The listing builds one solid part. Answer for the finished solid, in the listing's coordinates (mm). Give positions to 0.01 mm unless a question says otherwise; leave off trailing zeros. Loops run counter-clockwise (first coordinate to the right, second up) from the corner with the lowest first, then second, coordinate; pieces in that order, holes last. Notation, with made-up numbers: M -29,14 L -4,14 A10 cw -4,33 Z; hole C 67.5,43.5 d5. An arc over 180 degrees is marked long. Use one line per item in the form item = value. Start each with the question number.
1. Each of these flat-tipped pins is pushed along its axis until it touches: pin 1 Ø6 at (y, z) = (-17.5, -12.5) entering from +X; pin 2 Ø10 at (x, y) = (13, 18.5) entering from +Z; pin 3 Ø3 at (y, z) = (11, 4.5) entering from +X. Where does it stop, or does it pass through?
2. The part is cut by section A-A (y = 12). Write down the section's boundary in (x, z) (3 decimals).
3. Straight lines are drawn through the part: line 1 (Z direction, x = 4, y = 7); line 2 (Z direction, x = 0.5, y = 13); line 3 (X direction, y = -8.5, z = 14). For each, find the intervals that lie inside material, in ascending order. Write a range as from..to.
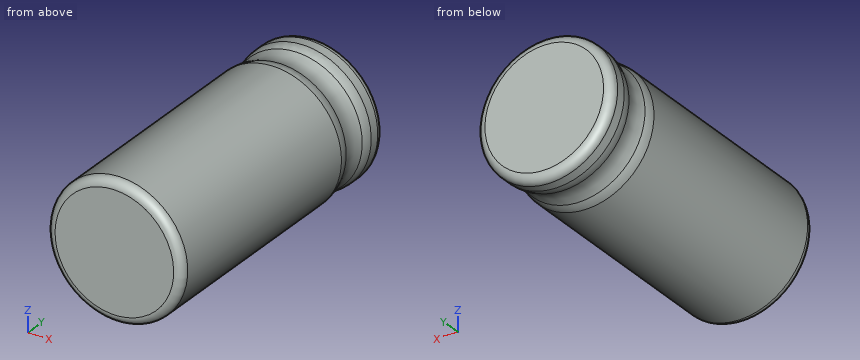
from build123d import *

# Parameters (mm, degrees)
SKETCH1_R           = 16.125
BOSS_EXTRUDE1_DEPTH = 35.25
FILLET1_R           = 2
FILLET2_R           = 6


with BuildPart() as part:
    # Sketch1 → Boss-Extrude1 (new, symmetric)
    with BuildSketch(Plane(origin=(0, 0, 0), x_dir=(1, 0, 0), z_dir=(0, 1, 0))):
        with Locations(Location((0, 0, 0), (0, 0, 270))):
            Circle(SKETCH1_R)
    extrude(amount=BOSS_EXTRUDE1_DEPTH, both=True)

    # Fillet1
    fillet1_edges = [part.edges().sort_by_distance(p)[0] for p in [
        (0, -35.25, -16.125),
        (0, 35.25, -16.125),
    ]]
    fillet(fillet1_edges, radius=FILLET1_R)

    # Sketch2 → Cut-Revolve1 (revolve, cut)
    with BuildSketch(Plane.XY, mode=Mode.PRIVATE) as cut_revolve1_sk:
        with BuildLine():
            ThreePointArc((16.125, 22), (15.035795209, 25.75), (16.125, 29.5))
            Line((16.125, 29.5), (16.125, 22))
        make_face()
    revolve(cut_revolve1_sk.sketch.rotate(Axis((0, 35.25, 0), (0, -1, 0)), 90), axis=Axis((0, 35.25, 0), (0, -1, 0)), mode=Mode.SUBTRACT)

    # Fillet2
    fillet2_edges = [part.edges().sort_by_distance(p)[0] for p in [
        (0, 29.5, -16.125),
        (0, 22, -16.125),
    ]]
    fillet(fillet2_edges, radius=FILLET2_R)


solid = part.part
Derived:
q1.pin_1 = 13.03
q1.pin_2 = 14
q1.pin_3 = 15.84
q2.outline = C 0,0 d32.25
q3.line_1 = -15.62..15.62
q3.line_2 = -16.12..16.12
q3.line_3 = -8..8
